Check sheet for the modelled part. Datum: model origin and axes. Units: mm. A direction names the side the tool comes from. Round coordinates to 2 decimals unless told otherwise and drop trailing zeros. Write each loop counter-clockwise with the first axis right and the second up, starting at its lowest first coordinate (ties: lowest second). Pieces come first, ordered by that corner, then holes. Notation, with made-up numbers: M 62,10 L 80,10 A30 cw 80,35 Z; hole C 87,39.5 d3. An arc over 180 degrees is marked long. Answer in a Markdown table with one row per item.
Autodesk Inventor part; units mm, degrees
ref_plane "YZ Plane" through (0, 0, 0) normal (1, 0, 0) x (0, 1, 0)
ref_plane "XZ Plane" through (0, 0, 0) normal (0, 1, 0) x (-1, 0, 0)
ref_plane "XY Plane" through (0, 0, 0) normal (0, 0, 1) x (1, 0, 0)
sketch "Sketch1" plane through (0, 0, 0) normal (0, 1, 0) x (-1, 0, 0)
  point P0 (0, 0)
sketch "Sketch2" plane through (0, 0, 0) normal (0, 1, 0) x (-1, 0, 0)
  line L0 (0, 0) -> (70, 0)
  line L1 (70, 0) -> (70, -66)
  line L2 (70, -66) -> (0, -66)
  line L3 (0, -66) -> (0, 0)
  dimension "d0" = 70
  dimension "d1" = 66
extrude "Extrusion1" add sketch "Sketch2" along normal blind 16.75
sketch "Sketch3" plane through (0, 16.75, 0) normal (0, 1, 0) x (1, 0, 0)
  point P0 (0, 0)
sketch "Sketch4" plane through (0, 16.75, 0) normal (0, 1, 0) x (1, 0, 0)
  line L0 (0, 66) -> (-70, 66)
  line L1 (-30.4814, 66) -> (-28.4814, 66)
  line L2 (-28.4814, 66) -> (-28.4814, 64)
  line L3 (-70, 66) -> (-70, 0)
  line L4 (-70, 37.8423) -> (-70, 39.8423)
  line L5 (-70, 39.8423) -> (-68, 39.8423)
  line L6 (-70, 0) -> (0, 0)
  line L7 (-28.4814, 0) -> (-30.4814, 0)
  line L8 (-30.4814, 0) -> (-30.4814, 2)
  line L9 (0, 0) -> (0, 66)
  line L10 (0, 38.8423) -> (0, 36.8423)
  line L11 (0, 36.8423) -> (-2, 36.8423)
  line L12 (-2, 2) -> (-60, 2)
  line L13 (-2, 64) -> (-2, 2)
  line L14 (-68, 64) -> (-68, 2)
  line L15 (-68, 64) -> (-2, 64)
  line L16 (-68, 2) -> (-2, 2)
  dimension "d5" = 2
  dimension "d6" = 2
  dimension "d7" = 2
  dimension "d8" = 2
  dimension "d9" = 2
  dimension "d10" = 2
  dimension "d11" = 2
  dimension "d12" = 2
  dimension "d102" = 2
  dimension "d103" = 2
  dimension "d104" = 2
extrude "Extrusion2" cut sketch "Sketch4" against normal blind 14.75 contours L15 L13 L12 L16 L14
sketch "Sketch10" plane through (0, 2, 0) normal (0, 1, 0) x (1, 0, 0)
  line L0 (-2, 2) -> (-68, 2)
  line L1 (-31, 2) -> (-48, 2)
  line L2 (-48, 2) -> (-48, 5)
  line L3 (-48, 2) -> (-63, 2)
  line L4 (-63, 2) -> (-63, 5)
  line L5 (-63, 5) -> (-48, 5)
  line L6 (-48, 5) -> (-48, 2)
  line L7 (-22, 64) -> (-7, 64)
  line L8 (-7, 64) -> (-7, 61)
  line L9 (-7, 61) -> (-22, 61)
  line L10 (-22, 61) -> (-22, 64)
  line L11 (-68, 64) -> (-2, 64)
  line L12 (-68, 64) -> (-68, 2)
  line L13 (-63, 2) -> (-48, 2)
  point P0 (-48, 5)
  point P1 (-63, 2)
  point P2 (-48, 2)
  dimension "d55" = 3
  dimension "d56" = 15
  dimension "d60" = 15
  dimension "d108" = 3
extrude "Extrusion5" add sketch "Sketch10" along normal blind 6
sketch "Sketch12" plane through (0, 0, 0) normal (0, -1, 0) x (1, 0, 0)
  line L0 (0, 0) -> (0, -66)
  arc A0 (-33, -49.6675) -> (-33, -42.7393) centre (-35, -46.2034) ccw
  arc A1 (-37, -52.3532) -> (-33, -52.3532) centre (-35, -52.3532) ccw
  line L1 (-33, -52.3532) -> (-33, -49.6675)
  line L2 (-37, -52.3532) -> (-37, -49.6675)
  arc A2 (-33, -42.7393) -> (-37, -49.6675) centre (-35, -46.2034) ccw
extrude "Extrusion7" cut sketch "Sketch12" against normal blind 5
sketch "Sketch13" plane through (0, 16.75, 0) normal (0, 1, 0) x (1, 0, 0)
  line L0 (-70, 66) -> (-70, 0)
  line L1 (0, 0) -> (0, 66)
  line L2 (-69, 1) -> (-1, 1)
  line L3 (-1, 1) -> (-1, 65)
  line L4 (-1, 65) -> (-69, 65)
  line L5 (-69, 65) -> (-69, 1)
  line L6 (-70, 0) -> (0, 0)
  line L7 (0, 66) -> (-70, 66)
  line L8 (-68, 64) -> (-2, 64)
  line L9 (-2, 64) -> (-2, 2)
  line L10 (-2, 2) -> (-68, 2)
  line L11 (-68, 2) -> (-68, 64)
  dimension "d94" = 1
  dimension "d95" = 1
  dimension "d96" = 1
  dimension "d97" = 1
  dimension "d98" = 1
  dimension "d99" = 1
  dimension "d100" = 1
  dimension "d101" = 1
extrude "Extrusion8" cut sketch "Sketch13" against normal blind 2 contours L5 L4 L3 L2 | L8 L9 L10 L11
sketch "Sketch15" plane through (-70, 0, -66) normal (-1, 0, 0) x (0, 0, 1)
  line L0 (62.4242, 8) -> (52.7396, 8)
  line L1 (0, 0) -> (66, 0)
  line L2 (0, 16.75) -> (66, 16.75)
  line L3 (0, 0) -> (0, 16.75)
  line L4 (16, 13.25) -> (25, 13.25)
  line L5 (25, 13.25) -> (25, 18.25)
  line L6 (25, 18.25) -> (16, 18.25)
  line L7 (16, 18.25) -> (16, 13.25)
  dimension "d118" = 8
  dimension "d140" = 25
  dimension "d141" = 9
  dimension "d142" = 3.5
  dimension "d143" = 5
extrude "Extrusion9" cut sketch "Sketch15" against normal blind 10
sketch "Sketch16" plane through (0, 0, -66) normal (0, 0, -1) x (-1, 0, 0)
  line L0 (41.4, 16.8) -> (49.9, 16.8)
  line L1 (49.9, 16.8) -> (49.9, 13.3)
  line L2 (49.9, 13.3) -> (41.4, 13.3)
  line L3 (41.4, 13.3) -> (41.4, 16.8)
  line L4 (56.5, 16.8) -> (65, 16.8)
  line L5 (65, 16.8) -> (65, 13.3)
  line L6 (65, 13.3) -> (56.5, 13.3)
  line L7 (56.5, 13.3) -> (56.5, 16.8)
  line L8 (22, 8) -> (7, 8)
  line L9 (70, 0) -> (70, 16.75)
  point P0 (0, 0)
  dimension "d127" = 8.5
  dimension "d128" = 8.5
  dimension "d129" = 3.5
  dimension "d130" = 5.3
  dimension "d131" = 28.6
  dimension "d132" = 13.5
extrude "Extrusion10" cut sketch "Sketch16" against normal blind 10
fillet "Fillet7" radius 2 1 edges at (0, 8.375, -66)
fillet "Fillet8" radius 2 1 edges at (-70, 8.375, -66)
properties part number "Shell 2 bottom"
1. Go/stop test with flat-tipped pins: pin 1 (2 mm diameter, centred on x = -62.5, z = -65, fed in from +Y); pin 2 (0.6 mm diameter, centred on y = 14.5, z = -65, fed in from -X); pin 3 (8 mm diameter, centred on x = -14.5, z = -53.5, fed in from +Y). Record where each tip stops, or that it passes through.
Found:
| item | result |
|---|---|
| pin 1 | stops at y = 13.3 |
| pin 2 | stops at x = -69.87 |
| pin 3 | stops at y = 2 |
2. Section check C-C, the plane z = -48. Record the cut outline in (x, y).
Found:
| item | result |
|---|---|
| outline | M -70,0 L -38.57,0 L -38.57,2 L -68,2 L -68,13.25 L -70,13.25 Z; M -31.43,0 L 0,0 L 0,16.75 L -1,16.75 L -1,14.75 L -2,14.75 L -2,2 L -31.43,2 Z |
3. Section check A-A, the plane x = -35. Record the cut outline in (y, z).
Found:
| item | result |
|---|---|
| outline | M 0,-66 L 16.75,-66 L 16.75,-65 L 14.75,-65 L 14.75,-64 L 2,-64 L 2,-54.35 L 0,-54.35 Z; M 0,-42.2 L 2,-42.2 L 2,-2 L 14.75,-2 L 14.75,-1 L 16.75,-1 L 16.75,0 L 0,0 Z |
4. Access from +Z, -Z, +X, -X, +Y, -Y to the whole of each face (thin tool, end or side, straight path). Record for faces 5 (the face through (-35, 8, 0)), 6 (the face through (-67, 16, -65)), 7 (the face through (-56.5, 14.6, -65.2)), 8 (the face through (-69.2, 14.6, -41)).
Found:
| item | result |
|---|---|
| face 5 | +Z, +X, -X, +Y, -Y |
| face 6 | +Y |
| face 7 | -Z, +Y |
| face 8 | -X, +Y |
5. Section check D-D, the plane x = -6. Record the cut outline in (y, z), and give its area (3 significant figures).
Found:
| item | result |
|---|---|
| outline | M 0,-66 L 16.75,-66 L 16.75,-65 L 14.75,-65 L 14.75,-64 L 2,-64 L 2,-2 L 14.75,-2 L 14.75,-1 L 16.75,-1 L 16.75,0 L 0,0 Z |
| area | 187 mm2 |
6. Scan lines: L1, parallel to Z at x = -35, y = 1.45; L2, parallel to X at y = 4.5, z = -50; L3, parallel to Z at x = -67, y = 12.25. Record each from-to range of solid material in increasing order.
Found:
| item | result |
|---|---|
| L1 | z = -66 to -54.35, -42.2 to 0 |
| L2 | x = -70 to -68, -2 to 0 |
| L3 | z = -66 to -64, -2 to 0 |
7. Section check B-B, the plane y = 11. Record the cut outline in (x, z), and give its area (3 significant figures).
Found:
| item | result |
|---|---|
| outline | M -70,-64 A2 ccw -68,-66 L -2,-66 A2 ccw 0,-64 L 0,0 L -70,0 Z; hole M -68,-64 L -2,-64 L -2,-2 L -68,-2 Z |
| area | 526 mm2 |
8. Draft check along X on faces 1 (the face through (-35, 16, -1)), 2 (the face through (-35, 0, -33)), 3 (the face through (-35.044, 0.986, -54.353)), 4 (the face through (-0.57, 8.49, -65.4)). Enter one of: +X half, -X half, draft (parallel to the pull), parting line (faces both ways), or undercut.
Found:
| item | result |
|---|---|
| face 1 | undercut |
| face 2 | draft |
| face 3 | undercut |
| face 4 | +X half |
